Here's how the part is built. I have some questions about the finished solid (model axes, mm). A direction names the side the tool comes from. Give positions to 0.01 mm unless a question says otherwise; leave off trailing zeros. Loops run counter-clockwise (first coordinate to the right, second up) from the corner with the lowest first, then second, coordinate; pieces in that order, holes last.
Q1. I'm going to push flat-ended pins straight in: P1, Ø5, axis at x = 3, z = -45.5, coming from the +Y side; P2, Ø16, axis at x = -4.5, y = 15.5, coming from the -Z side; P3, Ø5.5, axis at y = 17, z = -158, coming from the -X side. Where does each tip first touch, or does it pass through?
Q2. I need wall thicknesses on probe 1 along Z at (x, y) = (40.5, 19.5); probe 2 along Y at (x, z) = (24, -145); probe 3 along Z at (x, y) = (9.5, 14). Which ranges of each line are inside material? Lowest first, please.
Q3. Suppose I cut it at A-A (x = 42). List the corners of the cut face in (y, z) for me.
Q4. Suppose I cut it at C-C (z = -31.5). List the corners of the cut face in (x, y) for me, and give its area (3 significant figures).
Q5. Suppose I cut it at D-D (x = -31). List the corners of the cut face in (y, z) for me.
Q6. Suppose I cut it at B-B (y = 12.5). List the corners of the cut face in (x, z) for me.
Q7. For faces 1 (the face through (15.763, 15, -158)), 2 (the face through (31, 15, -155)), 3 (the face through (-1, -12, -5)), which set-ups out of +Z, -Z, +X, -X, +Y, -Y let a thin tool reach every point of the face, with its end or its side?
```python
from build123d import *

# Parameters (mm, degrees)
SKETCH1_W           = 100
SKETCH1_H           = 160
BOSS_EXTRUDE1_DEPTH = 5
SKETCH2_W           = 100
SKETCH2_H           = 50
BOSS_EXTRUDE2_DEPTH = 5
SKETCH4_W           = 160
SKETCH4_H           = 25
BOSS_EXTRUDE3_DEPTH = 5
SKETCH5_W           = 34.236688448
SKETCH5_H           = 25
BOSS_EXTRUDE4_DEPTH = 5


with BuildPart() as part:
    # Sketch1 → Boss-Extrude1 (new body)
    with BuildSketch(Plane(origin=(0, 0, 0), x_dir=(1, 0, 0), z_dir=(0, 1, 0))):
        with Locations((0, 80)):
            Rectangle(SKETCH1_W, SKETCH1_H)
    extrude(amount=BOSS_EXTRUDE1_DEPTH)

    # Sketch2 → Boss-Extrude2 (add)
    with BuildSketch(Plane.XY):
        Rectangle(SKETCH2_W, SKETCH2_H)
    extrude(amount=-BOSS_EXTRUDE2_DEPTH)

    # Sketch4 → Boss-Extrude3 (add)
    with BuildSketch(Plane(origin=(50, 0, 0), x_dir=(0, 0, -1), z_dir=(1, 0, 0))):
        with Locations((80, 12.5)):
            Rectangle(SKETCH4_W, SKETCH4_H)
    extrude(amount=-BOSS_EXTRUDE3_DEPTH)

    # Sketch5 → Boss-Extrude4 (add)
    with BuildSketch(Plane(origin=(0, 0, -160), x_dir=(-1, 0, 0), z_dir=(0, 0, -1))):
        with Locations((-32.881655776, 12.5)):
            Rectangle(SKETCH5_W, SKETCH5_H)
    extrude(amount=-BOSS_EXTRUDE4_DEPTH)


solid = part.part
```
Solutions:
1. P1: stops at y = 5
1. P2: stops at z = -5
1. P3: stops at x = 15.76
2. probe 1: z = -160 to -155, -5 to 0
2. probe 2: y = 0 to 5
2. probe 3: z = -5 to 0
3. outline: (-25, -5) - (0, -5) - (0, -160) - (25, -160) - (25, -155) - (5, -155) - (5, -5) - (25, -5) - (25, 0) - (-25, 0) - close
4. outline: (-50, 0) - (50, 0) - (50, 25) - (45, 25) - (45, 5) - (-50, 5) - close
4. area: 600 mm2
5. outline: (-25, -5) - (0, -5) - (0, -160) - (5, -160) - (5, -5) - (25, -5) - (25, 0) - (-25, 0) - close
6. outline: (-50, -5) - (45, -5) - (45, -155) - (15.76, -155) - (15.76, -160) - (50, -160) - (50, 0) - (-50, 0) - close
7. face 1: -Z, -X, +Y
7. face 2: -X, +Y
7. face 3: -Z, +X, -X, -Y
